from build123d import *

# Parameters (mm, degrees)
SKETCH1_W                = 11.43
SKETCH1_H                = 12.7
BOSS_EXTRUDE1_DEPTH      = 72.898
BOSS_EXTRUDE1_DEPTH_BACK = 72.898
SKETCH2_R                = 1.5875
BOSS_EXTRUDE2_DEPTH      = 4.7625
BOSS_EXTRUDE2_DEPTH_BACK = 4.7625
CUT_EXTRUDE1_DEPTH       = 1.6764
CUT_EXTRUDE1_DEPTH_BACK  = 1.6764


with BuildPart() as part:
    # Sketch1 → Boss-Extrude1 (new body, two sides)
    with BuildSketch(Plane.XY) as boss_extrude1_sk:
        with Locations((5.715, -6.35)):
            Rectangle(SKETCH1_W, SKETCH1_H)
    extrude(amount=BOSS_EXTRUDE1_DEPTH)
    extrude(boss_extrude1_sk.sketch, amount=-BOSS_EXTRUDE1_DEPTH_BACK)

    # Sketch2 → Boss-Extrude2 (add, two sides)
    with BuildSketch(Plane.XY) as boss_extrude2_sk:
        with BuildLine():
            Line((11.43, 0), (25.146, 0))
            ThreePointArc((25.146, 0), (28.917707571, -1.562292429), (30.48, -5.334))
            Line((30.48, -5.334), (30.48, -7.366))
            ThreePointArc((30.48, -7.366), (28.917707571, -11.137707571), (25.146, -12.7))
            Line((25.146, -12.7), (11.43, -12.7))
            Line((11.43, -12.7), (11.43, 0))
        make_face()
        with Locations((25.146, -6.35)):
            Circle(SKETCH2_R, mode=Mode.SUBTRACT)
    extrude(amount=BOSS_EXTRUDE2_DEPTH)
    extrude(boss_extrude2_sk.sketch, amount=-BOSS_EXTRUDE2_DEPTH_BACK)

    # Sketch3 → Cut-Extrude1 (cut, two sides)
    with BuildSketch(Plane.XY) as cut_extrude1_sk:
        with BuildLine():
            Line((11.43, 0), (11.43, -12.7))
            Line((11.43, -12.7), (25.146, -12.7))
            ThreePointArc((25.146, -12.7), (28.917707571, -11.137707571), (30.48, -7.366))
            Line((30.48, -7.366), (30.48, -5.334))
            ThreePointArc((30.48, -5.334), (28.917707571, -1.562292429), (25.146, 0))
            Line((25.146, 0), (11.43, 0))
        make_face()
    extrude(amount=CUT_EXTRUDE1_DEPTH, mode=Mode.SUBTRACT)
    extrude(cut_extrude1_sk.sketch, amount=-CUT_EXTRUDE1_DEPTH_BACK, mode=Mode.SUBTRACT)


solid = part.part
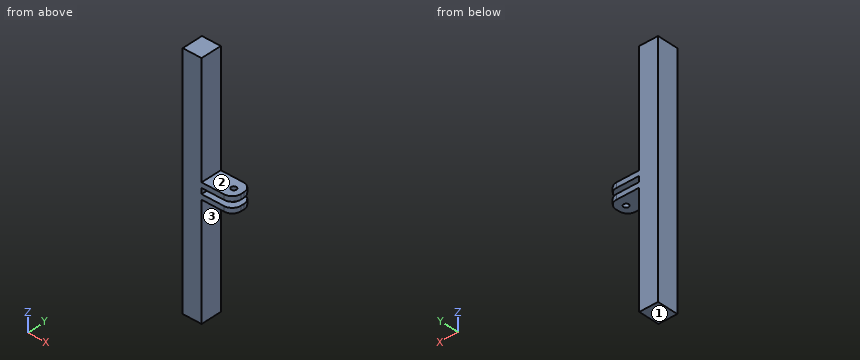
Could you check a few things on this model? Use its own coordinates, in mm. Face numbers are marked on the shaded views. A direction names the side the tool comes from. Coordinates: 2 decimals unless noted, no trailing zeros. Write each loop counter-clockwise with the first axis right and the second up, starting at its lowest first coordinate (ties: lowest second). Pieces come first, ordered by that corner, then holes. Notation, with made-up numbers: M 21,36 L 50,36 A15 cw 50,41 Z; hole C 77,8.25 d1. An arc over 180 degrees is marked long. One line per question, with ' | ' between items.
1) For the marked faces 1, 2 and 3, which set-ups out of +Z, -Z, +X, -X, +Y, -Y let a thin tool reach every point of the face, with its end or its side?
Checks:
face 1: -Z, +X, -X, +Y, -Y | face 2: +Z, +X, +Y, -Y | face 3: -Z, +X, +Y, -Y
2) For pin 1 Ø4 at (x, y) = (26, -2) entering from +Z; pin 2 Ø1 at (y, z) = (-8.5, 0.5) entering from +X, each with a flat end and sliding along its axis, tell me the tip position at first contact or that it passes through.
Checks:
pin 1: z = 4.76 | pin 2: x = 11.43
3) Imagine slicing it at C-C, the plane z = 29. Write out the boundary of the cut face in (x, y), and give its area (3 significant figures).
Checks:
outline: M 0,-12.7 L 11.43,-12.7 L 11.43,0 L 0,0 Z | area: 145 mm²
4) Imagine slicing it at B-B, the plane y = -10. Write out the boundary of the cut face in (x, z), and give its area (3 significant figures).
Checks:
outline: M 0,-72.9 L 11.43,-72.9 L 11.43,-4.76 L 29.78,-4.76 L 29.78,-1.68 L 11.43,-1.68 L 11.43,1.68 L 29.78,1.68 L 29.78,4.76 L 11.43,4.76 L 11.43,72.9 L 0,72.9 Z | area: 1,780 mm²
5) I need wall thicknesses on probe 1 along Z at (x, y) = (14, -8.75); probe 2 along X at (y, z) = (-11.75, -62.5); probe 3 along Y at (x, z) = (28, -3). Which ranges of each line are inside material? Lowest first, please. Write a range as [from, to].
Checks:
probe 1: [-4.76, -1.68], [1.68, 4.76] | probe 2: [0, 11.43] | probe 3: [-11.87, -0.83]
6) Imagine slicing it at D-D, the plane y = -3. Write out the boundary of the cut face in (x, z).
Checks:
outline: M 0,-72.9 L 11.43,-72.9 L 11.43,-4.76 L 29.94,-4.76 L 29.94,-1.68 L 11.43,-1.68 L 11.43,1.68 L 29.94,1.68 L 29.94,4.76 L 11.43,4.76 L 11.43,72.9 L 0,72.9 Z
